Work out the finished part from the listing and answer in its coordinate system (mm). Coordinates: 2 decimals unless noted, no trailing zeros. Loops run counter-clockwise (first coordinate to the right, second up) from the corner with the lowest first, then second, coordinate; pieces in that order, holes last. Notation, with made-up numbers: (32, 3.25) - (79, 3.25) arc R33 ccw to (79, 39.25) - close; hole circle Ø2 at (89.25, 89.5). An arc over 180 degrees is marked (long way). Write each question's results on one line, items separated by ' | '. Start each with the question number.
Item 1: Section B-B, the plane z = 1 is taken. Count the separate pieces of the cut face and the enclosed holes in it, plus the area to 3 significant figures.
Item 2: Section D-D, the plane y = 20 is taken. Write down the section's boundary in (x, z).
Item 3: Section C-C, the plane x = 188 is taken. Write down the section's boundary in (y, z), plus the area to 3 significant figures.
Item 4: Section A-A, the plane y = 0 is taken. Write down the section's boundary in (x, z).
Item 5: Consider probe 1 along X at (y, z) = (-1.5, 3.5); probe 2 along Y at (x, z) = (402.59, 4.5); probe 3 along X at (y, z) = (13, 1.5). Determine where each line is inside the solid, lowest interval first. Write a range as [from, to].
Item 6: This flat-tipped pin is pushed along its axis until it touches: pin 1 Ø1 at (x, z) = (170.5, 3) entering from -Y. Where does it stop, or does it pass through?
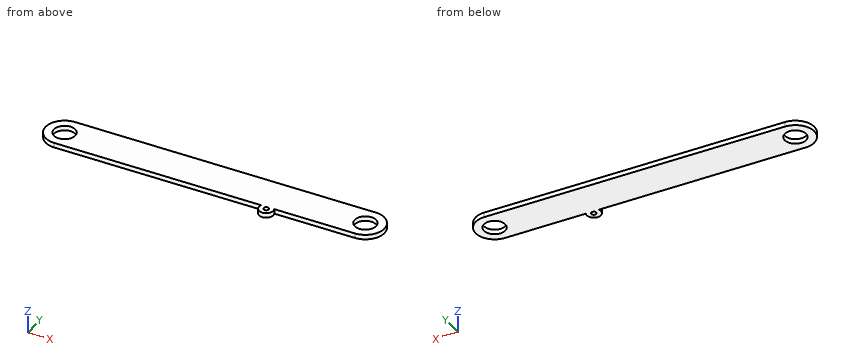
Autodesk Inventor part; units mm, degrees
ref_plane "YZ Plane" through (0, 0, 0) normal (1, 0, 0) x (0, 1, 0)
ref_plane "XZ Plane" through (0, 0, 0) normal (0, 1, 0) x (-1, 0, 0)
ref_plane "XY Plane" through (0, 0, 0) normal (0, 0, 1) x (1, 0, 0)
sketch "Sketch1" plane through (0, 0, 0) normal (0, 0, 1) x (1, 0, 0)
  circle A0 centre (0, 0) radius 14.2875
  circle A1 centre (402.59, 0) radius 14.2875
  line L0 (0, 0) -> (402.59, 0) construction
  line L1 (0, 0) -> (402.59, 0) construction
  line L2 (402.59, 25.4) -> (0, 25.4)
  arc A2 (0, 25.4) -> (0, -25.4) centre (0, 0) ccw
  arc A3 (402.59, -25.4) -> (402.59, 25.4) centre (402.59, 0) ccw
  arc A4 (276.9873, -25.4) -> (294.5127, -25.4) centre (285.75, -29.1338) ccw
  line L3 (0, -25.4) -> (276.9873, -25.4)
  line L4 (294.5127, -25.4) -> (402.59, -25.4)
  point P0 (201.295, 0)
  dimension "d0" = 28.575
  dimension "d1" = 402.59
  dimension "d2" = 50.8
  dimension "d3" = 285.75
  dimension "d15" = 29.1338
  dimension "d16" = 19.05
extrude "Extrusion1" add sketch "Sketch1" along normal blind 6.35
hole "Hole1" at (285.75, -29.1338, 0) direction (0, 0, 1) diameter 6.7564 end through all
properties part number "GP4-003" material "Aluminum 6061"
Answer key:
1) separate pieces: 1 | enclosed holes: 3 | area: 21,400 mm^2
2) outline: (-15.66, 0) - (418.25, 0) - (418.25, 6.35) - (-15.66, 6.35) - close
3) outline: (-25.4, 0) - (25.4, 0) - (25.4, 6.35) - (-25.4, 6.35) - close | area: 323 mm^2
4) outline: (-25.4, 0) - (-14.29, 0) - (-14.29, 6.35) - (-25.4, 6.35) - close; (14.29, 0) - (388.3, 0) - (388.3, 6.35) - (14.29, 6.35) - close; (416.88, 0) - (427.99, 0) - (427.99, 6.35) - (416.88, 6.35) - close
5) probe 1: x = [-25.36, -14.21], [14.21, 388.38], [416.8, 427.95] | probe 2: y = [-25.4, -14.29], [14.29, 25.4] | probe 3: x = [-21.82, -5.93], [5.93, 396.66], [408.52, 424.41]
6) pin 1: stops at y = -25.4
